For this review, take the finished solid that the model builds, in its own axes (mm). Face numbers are marked on the shaded views. A direction names the side the tool comes from. Coordinates: 2 decimals unless noted, no trailing zeros. Order: outer loops, then holes, each group sorted by start corner. A loop starts at its lowest first (then second) coordinate and runs counter-clockwise, first axis right, second up. Notation, with made-up numbers: M -38.75,59 L 15.25,59 A25 cw 15.25,86 Z; hole C 82.25,60.25 d2. An arc over 180 degrees is marked long. Use CSV: the item, a comma, the result in double quotes.
```python
from build123d import *

# Parameters (mm, degrees)
F0_R     = 26
F1_DEPTH = 15
F4_R     = 5


with BuildPart() as f1:
    # F0 (on Top) → F1 (new body)
    with BuildSketch(Plane.XY):
        Circle(F0_R)
    extrude(amount=F1_DEPTH)

    # F2 (on Right) → F3 (revolve)
    with BuildSketch(Plane.YZ):
        with BuildLine():
            Line((-45, 15), (0, 15))
            Line((0, 15), (0, 35))
            ThreePointArc((0, 35), (-23.504386, 30.513157), (-45, 20))
            Line((-45, 20), (-45, 15))
        make_face()
    revolve(axis=Axis((0, 0, 37.347408), (0, 0, 1)))

    # F4
    f4_edges = [f1.edges().sort_by_distance(p)[0] for p in [
        (0, 45, 20),
    ]]
    fillet(f4_edges, radius=F4_R)


solid = f1.part
```
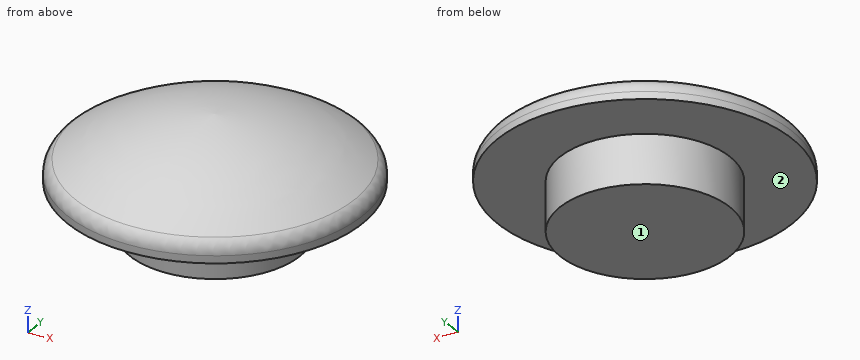
Item 1: Add section A-A on z = 2. State the section outline as (x, y) points, and give its area (3 significant figures).
Solutions:
outline,"C 0,0 d52"
area,"2,120 mm^2"
Item 2: For the marked faces 1 and 2, list the 3-axis set-ups (+Z, -Z, +X, -X, +Y, -Y) from which the entire face can be reached by the end or side of a thin tool; tool diameter is ignored.
Solutions:
face 1,"-Z, +X, -X, +Y, -Y"
face 2,"-Z"
Item 3: To check wall thickness, follow line 1 along Y through (x, z) = (0.5, 7); line 2 along X through (y, z) = (-31.5, 18); line 3 along Z through (x, y) = (17, 14.5). State the ranges of each line that lie inside material, in increasing order. Write a range as [from, to].
Solutions:
line 1,"[-26, 26]"
line 2,"[-32.06, 32.06]"
line 3,"[0, 30.89]"
Item 4: Clearance check with flat-ended pins moving along their axes: pin 1 Ø12 at (x, y) = (27, -32.5) entering from -Z; pin 2 Ø8 at (y, z) = (16.5, 10) entering from +X; pin 3 Ø10 at (y, z) = (-7.5, 16.5) entering from -X. State where each tip first meets the part, or that it passes through.
Solutions:
pin 1,"z = 15"
pin 2,"x = 22.8"
pin 3,"x = -44.93"
